from build123d import *

# Parameters (mm, degrees)
SKETCH_1_R          = 11.75
EXTRUDE_1_DEPTH     = 24.5
SKETCH_2_R          = 0.75
EXTRUDE_2_DEPTH     = 5
FILLET_1_R          = 0.75
SKETCH_3_R          = 7.4
CUT_EXTRUDE_1_DEPTH = 1.5
SKETCH_5_R          = 0.5


with BuildPart() as part:
    # 草图1 → 凸台-拉伸1 (new body)
    with BuildSketch(Plane.XY):
        Circle(SKETCH_1_R)
    extrude(amount=EXTRUDE_1_DEPTH)

    # 草图2 → 凸台-拉伸2 (add)
    with BuildSketch(Plane.XY.offset(24.5)):
        with Locations((-6.408587988, 3.7)):
            Circle(SKETCH_2_R)
        with Locations((0, 7.4)):
            Circle(SKETCH_2_R)
        with Locations((6.408587988, 3.7)):
            Circle(SKETCH_2_R)
        with Locations((6.408587988, -3.7)):
            Circle(SKETCH_2_R)
        with Locations((-6.408587988, -3.7)):
            Circle(SKETCH_2_R)
    extrude(amount=EXTRUDE_2_DEPTH)

    # 圆角1
    fillet_1_edges = [part.edges().sort_by_distance(p)[0] for p in [
        (5.658587988, 3.7, 29.5),
        (5.658587988, -3.7, 29.5),
        (-7.158587988, -3.7, 29.5),
        (-7.158587988, 3.7, 29.5),
        (-0.75, 7.4, 29.5),
    ]]
    fillet(fillet_1_edges, radius=FILLET_1_R)

    # 草图3 → 切除-拉伸1 (cut)
    with BuildSketch(Plane(origin=(0, 0, 0), x_dir=(-1, 0, 0), z_dir=(0, 0, -1))):
        Circle(SKETCH_3_R)
    extrude(amount=-CUT_EXTRUDE_1_DEPTH, mode=Mode.SUBTRACT)

    # 扫描1: sweep along a path in 草图4
    with BuildLine(Plane(origin=(0, 0, 0), x_dir=(-1, 0, 0), z_dir=(0, 0, -1))) as sweep_1_path:
        CenterArc((0, 0), 9.575, 0, 360)
    # 草图5 → 扫描1 (sweep)
    with BuildSketch(Plane(origin=(0, 0, 0), x_dir=(1, 0, 0), z_dir=(0, 1, 0))):
        with Locations((-9.575, 0)):
            Circle(SKETCH_5_R)
    sweep(path=sweep_1_path.line)


solid = part.part
Can you work these out from the model? Positions are in its coordinate system, mm. A direction names the side the tool comes from. Coordinates: 2 decimals unless noted, no trailing zeros. Write each loop counter-clockwise with the first axis right and the second up, starting at its lowest first coordinate (ties: lowest second). Pieces come first, ordered by that corner, then holes. Notation, with made-up numbers: (-18, 25) - (-13, 25) arc R23 ccw to (-13, 40) - close; hole circle Ø3 at (-18.5, 43). An arc over 180 degrees is marked (long way). Return JSON: item names as keys, results as strings. Group by question number.
Item 1: If we section it at B-B (x = 0): Write out the boundary of the cut face in (y, z) (3 decimals).
Item 2: If we section it at C-C (z = 26.5): Write out the boundary of the cut face in (x, y).
Item 3: I'm going to push flat-ended pins straight in: pin 1 Ø10 at (x, z) = (-9.5, 22.5) entering from +Y; pin 2 Ø1.5 at (y, z) = (-9, 5) entering from +X; pin 3 Ø6 at (x, z) = (9.5, 18.5) entering from +Y. Where does each tip first touch, or does it pass through?
Item 4: If we section it at D-D (x = 10.5): Write out the boundary of the cut face in (y, z), then the cut area to 3 significant figures.
Item 5: Please list where these lines run through material, in increasing order: probe 1 along Y at (x, z) = (0, 0.45); probe 2 along Z at (x, y) = (-4, -1.5); probe 3 along Z at (x, y) = (-3.75, -7).
Item 6: We'd pull the mould along Y, two halves only. Please class faces 4 (the face through (-5.693, -3.475, 26.595)), 5 (the face through (5, 9, 0)), 6 (the face through (-0.163, 6.668, 26.595)): pulls with the +Y half, pulls with the -Y half, needs draft (parallel to the pull), parting line crosses it, or undercut.
Item 7: If we section it at A-A (y = 0): Write out the boundary of the cut face in (x, z) (3 decimals).
Item 8: Which directions (+Z, -Z, +X, -X, +Y, -Y) give clear straight access to the entire face, cutting with the end or side of a thin tool? Please do faces 1 (the face through (-5.693, 3.925, 26.595)), 2 (the face through (11.207, 3.529, 12.078)), 3 (the face through (1.604, -7.224, 0.74)).
Return value:
{
 "1": {"outline": "(-11.75, 0) - (-10.075, 0) arc R0.5 ccw to (-9.075, 0) - (-7.4, 0) - (-7.4, 1.5) - (7.4, 1.5) - (7.4, 0) - (9.075, 0) arc R0.5 ccw to (10.075, 0) - (11.75, 0) - (11.75, 24.5) - (8.15, 24.5) - (8.15, 28.75) arc R0.75 ccw to (6.65, 28.75) - (6.65, 24.5) - (-11.75, 24.5) - close"},
 "2": {"outline": "circle Ø1.5 at (-6.41, -3.7); circle Ø1.5 at (-6.41, 3.7); circle Ø1.5 at (0, 7.4); circle Ø1.5 at (6.41, -3.7); circle Ø1.5 at (6.41, 3.7)"},
 "3": {"pin 1": "stops at y = 10.85", "pin 2": "stops at x = 8.37", "pin 3": "stops at y = 9.79"},
 "4": {"outline": "(-5.27, 0) - (5.27, 0) - (5.27, 24.5) - (-5.27, 24.5) - close", "area": "258 mm^2"},
 "5": {"probe 1": "y = -11.75 to -7.4, 7.4 to 11.75", "probe 2": "z = 1.5 to 24.5", "probe 3": "z = 0 to 24.5"},
 "6": {"face 4": "undercut", "face 5": "needs draft", "face 6": "parting line crosses it"},
 "7": {"outline": "(-11.75, 0) - (-10.075, 0) arc R0.5 ccw to (-9.075, 0) - (-7.4, 0) - (-7.4, 1.5) - (7.4, 1.5) - (7.4, 0) - (9.075, 0) arc R0.5 ccw to (10.075, 0) - (11.75, 0) - (11.75, 24.5) - (-11.75, 24.5) - close"},
 "8": {"face 1": "+Z", "face 2": "+Z, -Z", "face 3": "-Z"}
}
